Design review of the part built by this model. Coordinates are the model's own, in mm. A direction names the side the tool comes from. Coordinates: 2 decimals unless noted, no trailing zeros. Loops run counter-clockwise (first coordinate to the right, second up) from the corner with the lowest first, then second, coordinate; pieces in that order, holes last. Notation, with made-up numbers: (-36, 24) -> (-31, 24) arc R20 cw to (-31, 61) -> close; hole circle Ø6 at (51.25, 62.25). An arc over 180 degrees is marked (long way). Answer as a JSON object with one key per item and string values.
```python
from build123d import *

# Parameters (mm, degrees)
EXTRUDE_1_DEPTH     = 7
SKETCH_12_R         = 1.5
CUT_EXTRUDE_1_DEPTH = 12
SKETCH_13_R         = 1.5
CUT_EXTRUDE_2_DEPTH = 12
SKETCH_14_R         = 1.5
CUT_EXTRUDE_3_DEPTH = 12
CUT_EXTRUDE_4_DEPTH = 8
CUT_EXTRUDE_5_DEPTH = 2.2
CUT_EXTRUDE_6_DEPTH = 5.8


with BuildPart() as part:
    # 草圖1 → 填料-伸長1 (new body)
    with BuildSketch(Plane.XY):
        Polygon((-22.5, 63), (22.5, 63), (65.809600438, -12.014428415), (43.309600438, -50.985571585), (-43.309600438, -50.985571585), (-65.809600438, -12.014428415), align=None)
    extrude(amount=EXTRUDE_1_DEPTH)

    # 草圖12 → 除料-伸長1 (cut)
    with BuildSketch(Plane(origin=(-54.559600438, -31.5, 0), x_dir=(0, 0, 1), z_dir=(-0.866025404, -0.5, 0))):
        with Locations((3.5, 15)):
            Circle(SKETCH_12_R)
        with Locations((3.5, -15)):
            Circle(SKETCH_12_R)
    extrude(amount=-CUT_EXTRUDE_1_DEPTH, mode=Mode.SUBTRACT)

    # 草圖13 → 除料-伸長2 (cut)
    with BuildSketch(Plane(origin=(54.559600438, -31.5, 0), x_dir=(0, 0, -1), z_dir=(0.866025404, -0.5, 0))):
        with Locations((-3.5, 15)):
            Circle(SKETCH_13_R)
        with Locations((-3.5, -15)):
            Circle(SKETCH_13_R)
    extrude(amount=-CUT_EXTRUDE_2_DEPTH, mode=Mode.SUBTRACT)

    # 草圖14 → 除料-伸長3 (cut)
    with BuildSketch(Plane(origin=(0, 63, 0), x_dir=(1, 0, 0), z_dir=(0, 1, 0))):
        with Locations((-15, -3.5)):
            Circle(SKETCH_14_R)
        with Locations((15, -3.5)):
            Circle(SKETCH_14_R)
    extrude(amount=-CUT_EXTRUDE_3_DEPTH, mode=Mode.SUBTRACT)

    # 草圖15 → 除料-伸長4 (cut, through all)
    with BuildSketch(Plane.XY.offset(7)):
        Polygon((31.762595055, -30.985571585), (42.715589671, -12.014428415), (10.952994616, 43), (-10.952994616, 43), (-42.715589671, -12.014428415), (-31.762595055, -30.985571585), align=None)
    extrude(amount=-CUT_EXTRUDE_4_DEPTH, mode=Mode.SUBTRACT)

    # 草圖16 → 除料-伸長5 (cut)
    with BuildSketch(Plane.XY.offset(7)):
        Polygon((41.114092363, -14.788303121), (54.104473419, -22.288303121), (46.354473419, -35.711696879), (33.364092363, -28.211696879), align=None)
    extrude(amount=-CUT_EXTRUDE_5_DEPTH, mode=Mode.SUBTRACT)

    # 草圖17 → 除料-伸長6 (cut, through all)
    with BuildSketch(Plane.XY.offset(4.8)):
        Polygon((41.114092363, -14.788303121), (39.714092363, -17.213174251), (52.704473419, -24.713174251), (54.104473419, -22.288303121), align=None)
    extrude(amount=-CUT_EXTRUDE_6_DEPTH, mode=Mode.SUBTRACT)


solid = part.part
```
1) The part is to be moulded in two halves that separate along X. For faces 1 (the flat face through (-44.458, 24.968, 3.451)), 2 (the flat face through (1, -50.986, 3)), 3 (the cylindrical face through (-16.5, 57.08, 3.43)), say which applies: pulls with the +X half, pulls with the -X half, needs draft (parallel to the pull), parting line crosses it, or undercut.
Completed:
{"face 1": "pulls with the -X half", "face 2": "needs draft", "face 3": "undercut"}
2) Wall thickness on probe 1 along Y at (x, z) = (-0.5, 4.75); probe 2 along X at (y, z) = (55.25, 3.5); probe 3 along Z at (x, y) = (-15, 54.5): over which ranges is each line inside the solid? List them lowest first.
Completed:
{"probe 1": "-50.99 to -30.99, 43 to 63", "probe 2": "-26.97 to -16.5, -13.5 to 13.5, 16.5 to 26.97", "probe 3": "0 to 2, 5 to 7"}
3) Add section C-C, the plane y = -32.5. Give the boundary of the cut face in (x, z).
Completed:
{"outline": "(-53.98, 0) -> (53.98, 0) -> (53.98, 7) -> (48.21, 7) -> (48.21, 4.8) -> (40.79, 4.8) -> (40.79, 7) -> (-53.98, 7) -> close"}
4) Clearance check with flat-ended pins moving along their axes: pin 1 Ø1 at (x, z) = (46.5, 5) entering from -Y; pin 2 Ø3.5 at (x, z) = (15.5, 3.5) entering from +Y; pin 3 Ø4 at (x, y) = (-11, 35) entering from +Z; pin 4 Ø2.5 at (x, z) = (15, 3.5) entering from +Y. State where each tip first meets the part, or that it passes through.
Completed:
{"pin 1": "y = -46.33", "pin 2": "y = 63", "pin 3": "through", "pin 4": "y = 51"}
5) Add section A-A, the plane x = -8. Give the boundary of the cut face in (y, z), and give its area (3 significant figures).
Completed:
{"outline": "(-50.99, 0) -> (-30.99, 0) -> (-30.99, 7) -> (-50.99, 7) -> close; (43, 0) -> (63, 0) -> (63, 7) -> (43, 7) -> close", "area": "280 mm²"}
6) Add section B-B, the plane y = 2. Give the boundary of the cut face in (x, z).
Completed:
{"outline": "(-57.72, 0) -> (-34.62, 0) -> (-34.62, 7) -> (-57.72, 7) -> close; (34.62, 0) -> (57.72, 0) -> (57.72, 7) -> (34.62, 7) -> close"}
7) Add section D-D, the plane x = 15. Give the boundary of the cut face in (y, z).
Completed:
{"outline": "(-50.99, 0) -> (-30.99, 0) -> (-30.99, 7) -> (-50.99, 7) -> close; (35.99, 0) -> (63, 0) -> (63, 2) -> (51, 2) -> (51, 5) -> (63, 5) -> (63, 7) -> (35.99, 7) -> close"}
8) For faces 4 (the flat face through (47.7, -18.59, 3.55)), 5 (the cylindrical face through (57.16, -15.16, 2.07)), 6 (the flat face through (15, 51, 3)), 7 (the flat face through (43, -26, 4.8)), list the 3-axis set-ups (+Z, -Z, +X, -X, +Y, -Y) from which the entire face can be reached by the end or side of a thin tool; tool diameter is ignored.
Completed:
{"face 4": "+Z, -Z", "face 5": "none", "face 6": "+Y", "face 7": "+Z"}
